Read the model definition and answer for the solid it produces. Units are mm, in the model's axes. A direction names the side the tool comes from. Round coordinates to 2 decimals unless told otherwise and drop trailing zeros. Order: outer loops, then holes, each group sorted by start corner. A loop starts at its lowest first (then second) coordinate and runs counter-clockwise, first axis right, second up. Notation, with made-up numbers: (76, 56.25) -> (119, 56.25) arc R33 ccw to (119, 94.25) -> close; hole circle Ø11 at (-8, 74). An arc over 180 degrees is marked (long way). Answer as a JSON object with one key per item and string values. Group by question number.
Item 1: Consider probe 1 along Z at (x, y) = (-63.5, 4.5) (3 decimals); probe 2 along X at (y, z) = (3, 63.5) (3 decimals); probe 3 along Z at (x, y) = (-64, 6) (3 decimals). Determine where each line is inside the solid, lowest interval first. Write a range as from..to.
Item 2: Section A-A, the plane x = 63.5 is taken. Write down the section's boundary in (y, z) (3 decimals), plus the area to 3 significant figures.
Item 3: For faces 5 (the flat face through (-60.325, 3, 0)), 6 (the flat face through (73.025, 3, -43)), 7 (the flat face through (60.325, 3, 0)), determine the directions among +Z, -Z, +X, -X, +Y, -Y from which every point of the face is accessible in a straight line to the end or side of a thin tool.
Item 4: Section D-D, the plane z = -6 is taken. Write down the section's boundary in (x, y) (3 decimals), plus the area to 3 significant figures.
Item 5: Given P1, Ø3.5, axis at x = -63.5, z = -63.5, coming from the +Y side; P2, Ø3, axis at y = 3, z = -3.5, coming from the -X side (3 decimals), each flat-ended and moving along its own axis, determine where each tip first touches the part or whether it passes through.
Item 6: Section C-C, the plane y = 4.75 is taken. Write down the section's boundary in (x, z) (3 decimals), plus the area to 3 significant figures.
Item 7: Section B-B, the plane z = -63.5 is taken. Write down the section's boundary in (x, y) (3 decimals).
Item 8: The mould has two halves that part along X. Classify faces 1 (the flat face through (73.025, 3, 43)), 2 (the flat face through (-1, 0, -1)), 3 (the cylindrical face through (64.49, 3.22, 65.41)), 4 (the flat face through (-73.025, 3, 43)): pulls with the +X half, pulls with the -X half, needs draft (parallel to the pull), parting line crosses it, or undercut.
from build123d import *

# Parameters (mm, degrees)
SKETCH1_W           = 146.05
SKETCH1_H           = 146.05
BOSS_EXTRUDE1_DEPTH = 6.35
SKETCH2_R           = 2.15265
CUT_EXTRUDE1_DEPTH  = 6.35
FILLET1_R           = 6.35
SKETCH3_W           = 12.7
SKETCH3_H           = 38.1
CUT_EXTRUDE2_DEPTH  = 6.35


with BuildPart() as part:
    # Sketch1 → Boss-Extrude1 (new body)
    with BuildSketch(Plane(origin=(0, 0, 0), x_dir=(1, 0, 0), z_dir=(0, 1, 0))):
        Rectangle(SKETCH1_W, SKETCH1_H)
    extrude(amount=BOSS_EXTRUDE1_DEPTH)

    # Sketch2 → Cut-Extrude1 (cut)
    with BuildSketch(Plane(origin=(0, 6.35, 0), x_dir=(1, 0, 0), z_dir=(0, 1, 0))):
        with Locations((-63.5, 63.5)):
            Circle(SKETCH2_R)
        with Locations((63.5, 63.5)):
            Circle(SKETCH2_R)
        with Locations((63.5, -63.5)):
            Circle(SKETCH2_R)
        with Locations((-63.5, -63.5)):
            Circle(SKETCH2_R)
    extrude(amount=-CUT_EXTRUDE1_DEPTH, mode=Mode.SUBTRACT)

    # Fillet1
    fillet1_edges = [part.edges().sort_by_distance(p)[0] for p in [
        (73.025, 3.175, 73.025),
        (-73.025, 3.175, 73.025),
        (-73.025, 3.175, -73.025),
        (73.025, 3.175, -73.025),
    ]]
    fillet(fillet1_edges, radius=FILLET1_R)

    # Sketch3 → Cut-Extrude2 (cut)
    with BuildSketch(Plane(origin=(0, 6.35, 0), x_dir=(1, 0, 0), z_dir=(0, 1, 0))):
        with Locations((66.675, 0)):
            Rectangle(SKETCH3_W, SKETCH3_H)
    cut_extrude2 = extrude(amount=-CUT_EXTRUDE2_DEPTH, mode=Mode.SUBTRACT)

    # Mirror1: Cut-Extrude2 across plane
    add(cut_extrude2.mirror(Plane(origin=(0, 0, 0), x_dir=(0, 0, 1), z_dir=(1, 0, 0))), mode=Mode.SUBTRACT)


solid = part.part
Values found:
{
 "1": {"probe 1": "-73.025..-65.653, -61.347..-19.05, 19.05..61.347, 65.653..73.025", "probe 2": "-73.025..-65.653, -61.347..61.347, 65.653..73.025", "probe 3": "-73.025..-65.594, -61.406..-19.05, 19.05..61.406, 65.594..73.025"},
 "2": {"outline": "(0, -73.025) -> (6.35, -73.025) -> (6.35, -65.653) -> (0, -65.653) -> close; (0, -61.347) -> (6.35, -61.347) -> (6.35, -19.05) -> (0, -19.05) -> close; (0, 19.05) -> (6.35, 19.05) -> (6.35, 61.347) -> (0, 61.347) -> close; (0, 65.653) -> (6.35, 65.653) -> (6.35, 73.025) -> (0, 73.025) -> close", "area": "631 mm2"},
 "3": {"face 5": "-X, +Y, -Y", "face 6": "+Z, -Z, +X, +Y, -Y", "face 7": "+X, +Y, -Y"},
 "4": {"outline": "(-60.325, 0) -> (60.325, 0) -> (60.325, 6.35) -> (-60.325, 6.35) -> close", "area": "766 mm2"},
 "5": {"P1": "through", "P2": "x = -60.325"},
 "6": {"outline": "(-73.025, -66.675) arc R6.35 ccw to (-66.675, -73.025) -> (66.675, -73.025) arc R6.35 ccw to (73.025, -66.675) -> (73.025, -19.05) -> (60.325, -19.05) -> (60.325, 19.05) -> (73.025, 19.05) -> (73.025, 66.675) arc R6.35 ccw to (66.675, 73.025) -> (-66.675, 73.025) arc R6.35 ccw to (-73.025, 66.675) -> (-73.025, 19.05) -> (-60.325, 19.05) -> (-60.325, -19.05) -> (-73.025, -19.05) -> close; hole circle Ø4.305 at (-63.5, -63.5); hole circle Ø4.305 at (-63.5, 63.5); hole circle Ø4.305 at (63.5, -63.5); hole circle Ø4.305 at (63.5, 63.5)", "area": "20,300 mm2"},
 "7": {"outline": "(-73.025, 0) -> (-65.653, 0) -> (-65.653, 6.35) -> (-73.025, 6.35) -> close; (-61.347, 0) -> (61.347, 0) -> (61.347, 6.35) -> (-61.347, 6.35) -> close; (65.653, 0) -> (73.025, 0) -> (73.025, 6.35) -> (65.653, 6.35) -> close"},
 "8": {"face 1": "pulls with the +X half", "face 2": "needs draft", "face 3": "undercut", "face 4": "pulls with the -X half"}
}
